For this review, take the finished solid that the model builds, in its own axes (mm). A direction names the side the tool comes from. Round coordinates to 2 decimals unless told otherwise and drop trailing zeros. Write each loop counter-clockwise with the first axis right and the second up, starting at its lowest first coordinate (ties: lowest second). Pieces come first, ordered by that corner, then holes. Notation, with made-up numbers: (15, -32) -> (52, -32) arc R17 ccw to (52, -26) -> close; hole circle Ø1 at (-7.75, 11.25). An arc over 180 degrees is marked (long way). Answer in a Markdown table with one row per item.
Autodesk Inventor part; units mm, degrees
ref_plane "YZ Plane" through (0, 0, 0) normal (1, 0, 0) x (0, 1, 0)
ref_plane "XZ Plane" through (0, 0, 0) normal (0, 1, 0) x (-1, 0, 0)
ref_plane "XY Plane" through (0, 0, 0) normal (0, 0, 1) x (1, 0, 0)
sketch "Sketch1" plane through (0, 0, 0) normal (0, 1, 0) x (-1, 0, 0)
  arc A0 (13, 0) -> (-13, 0) centre (0, 0) ccw
  circle A1 centre (0, 0) radius 1.25
  arc A2 (-4.9331, -48.8152) -> (4.9331, -48.8152) centre (0, -48) ccw
  line L0 (13, 0) -> (4.9331, -48.8152)
  line L1 (-13, 0) -> (-4.9331, -48.8152)
  circle A3 centre (0, -48) radius 1.25
  dimension "d3" = 2.5
  dimension "d16" = 10
  dimension "d17" = 2.5
  dimension "d19" = 13
  dimension "d20" = 48
extrude "Extrusion1" add sketch "Sketch1" along normal blind 4
sketch "Sketch2" plane through (0, 4, 0) normal (0, 1, 0) x (1, 0, 0)
  line L0 (-3, -13) -> (3, -13)
  line L1 (3, 13) -> (-3, 13)
  circle A0 centre (0, 0) radius 1.25
  line L2 (-3, -13) -> (3, 13) construction
  line L3 (3, -13) -> (-3, 13) construction
  line L4 (9, 1.7894) -> (9, -1.8106)
  line L5 (-9, -1.7894) -> (-9, 1.8106)
  line L6 (-9, 1.8106) -> (9, -1.8106) construction
  line L7 (9, 1.7894) -> (-9, -1.7894) construction
  line L8 (3, 1.7894) -> (9, 1.7894)
  line L9 (-9, 1.8106) -> (-3, 1.8106)
  line L10 (-3, -1.7894) -> (-9, -1.7894)
  line L11 (9, -1.8106) -> (3, -1.8106)
  line L12 (3, 1.7894) -> (3, 13)
  line L13 (3, -13) -> (3, -1.8106)
  line L14 (-3, -1.7894) -> (-3, -13)
  line L15 (-3, 13) -> (-3, 1.8106)
  point P0 (-9, 0.0106)
  dimension "d7" = 6
  dimension "d12" = 3.6
  dimension "d13" = 13
  dimension "d14" = 13
  dimension "d15" = 9
extrude "Extrusion2" cut sketch "Sketch2" against normal blind 2 contours L14 L10 L5 L9 L15 L1 L12 L8 L4 L11 L13 L0 | A0
fillet "Fillet3" radius 2 4 edges at (-3, 3, -1.8106) (-3, 3, 1.7894) (3, 3, -1.7894) (3, 3, 1.8106)
properties part number "6P-016"
1) Clearance check with flat-ended pins moving along their axes: pin 1 Ø0.6 at (y, z) = (3.5, -8) entering from -X; pin 2 Ø1 at (y, z) = (3.5, 1) entering from -X; pin 3 Ø1 at (y, z) = (3, 8.5) entering from +X. State where each tip first meets the part, or that it passes through.
Solved:
| item | result |
|---|---|
| pin 1 | x = -11.73 |
| pin 2 | x = -12.99 |
| pin 3 | x = 10.25 |
2) Consider section A-A on y = 3.1. State the section outline as (x, z) points.
Solved:
| item | result |
|---|---|
| outline | (-13, 0) -> (-4.93, -48.82) arc R5 ccw to (4.93, -48.82) -> (13, 0) arc R13 ccw to (3, 12.65) -> (3, 3.81) arc R2 ccw to (5, 1.81) -> (9, 1.81) -> (9, -1.79) -> (5, -1.79) arc R2 ccw to (3, -3.79) -> (3, -13) -> (-3, -13) -> (-3, -3.81) arc R2 ccw to (-5, -1.81) -> (-9, -1.81) -> (-9, 1.79) -> (-5, 1.79) arc R2 ccw to (-3, 3.79) -> (-3, 12.65) arc R13 ccw to start; hole circle Ø2.5 at (0, -48) |
3) For faces 4 (the flat face through (0, 0, -12)), 5 (the flat face through (-7, 3, -1.811)), 6 (the flat face through (-3, 3, 8)), list the 3-axis set-ups (+Z, -Z, +X, -X, +Y, -Y) from which the entire face can be reached by the end or side of a thin tool; tool diameter is ignored.
Solved:
| item | result |
|---|---|
| face 4 | +Z, -Z, +X, -X, -Y |
| face 5 | +Y |
| face 6 | +Z, +Y |
4) For line 1 (X direction, y = 0.55, z = 0); line 2 (X direction, y = 2.85, z = -8); line 3 (Y direction, x = 3.25, z = 1), list the stretches that pass through material, from the lowest coordinate up. Write a range as [from, to].
Solved:
| item | result |
|---|---|
| line 1 | [-13, -1.25], [1.25, 13] |
| line 2 | [-11.68, -3], [3, 11.68] |
| line 3 | [0, 2] |
5) Consider section C-C on z = -48. State the section outline as (x, y) points, then the cut area to 3 significant figures.
Solved:
| item | result |
|---|---|
| outline | (-5.07, 0) -> (-1.25, 0) -> (-1.25, 4) -> (-5.07, 4) -> close; (1.25, 0) -> (5.07, 0) -> (5.07, 4) -> (1.25, 4) -> close |
| area | 30.5 mm² |
6) Mouldability with a two-part tool opening along X and no side actions: class faces 1 (the flat face through (0, 4, -20)), 2 (the flat face through (9, 3, 0)), 3 (the cylindrical face through (0, 2, -53)) as pulls with the +X half, pulls with the -X half, needs draft (parallel to the pull), parting line crosses it, or undercut.
Solved:
| item | result |
|---|---|
| face 1 | needs draft |
| face 2 | undercut |
| face 3 | parting line crosses it |
7) Consider section D-D on z = 8. State the section outline as (x, y) points, then the cut area to 3 significant figures.
Solved:
| item | result |
|---|---|
| outline | (-10.25, 0) -> (10.25, 0) -> (10.25, 4) -> (3, 4) -> (3, 2) -> (-3, 2) -> (-3, 4) -> (-10.25, 4) -> close |
| area | 70.0 mm² |
8) Consider section B-B on x = 0. State the section outline as (y, z) points, then the cut area to 3 significant figures.
Solved:
| item | result |
|---|---|
| outline | (0, -53) -> (4, -53) -> (4, -49.25) -> (0, -49.25) -> close; (0, -46.75) -> (4, -46.75) -> (4, -13) -> (2, -13) -> (2, -1.25) -> (0, -1.25) -> close; (0, 1.25) -> (2, 1.25) -> (2, 13) -> (0, 13) -> close |
| area | 197 mm² |
